Autodesk Inventor part; units mm, degrees
ref_plane "Work Plane2" through (300, 100, 0) normal (-0.9889364, -0.1483405, 0) x (0.1483405, -0.9889364, 0)
ref_plane "YZ Plane" through (0, 0, 0) normal (1, 0, 0) x (0, 1, 0)
ref_plane "XZ Plane" through (0, 0, 0) normal (0, 1, 0) x (-1, 0, 0)
sketch "Sketch1" plane through (0, 0, 0) normal (0, 0, 1) x (1, 0, 0)
  line L0 (-100, 0) -> (100, 0) construction
  line L1 (-100, 65) -> (-100, -65)
  circle A0 centre (-52.5, 57.5) radius 2.25
  line L2 (100, -70) -> (100, 70) construction
  line L3 (-92, 0) -> (-92, 57.5) construction
  line L4 (-92, 0) -> (-92, -57.5) construction
  circle A1 centre (-92.5, 57.5) radius 2.25
  circle A2 centre (-92.5, 57.5) radius 1.25
  circle A3 centre (-52.5, 57.5) radius 1.25
  line L5 (-100, 65) -> (-22.5777, 65)
  line L6 (-22.5777, 65) -> (-12.5777, 90)
  line L7 (-12.5777, 90) -> (100, 90)
  line L8 (100, 90) -> (100, 0)
  line L9 (100, -90) -> (100, 0)
  line L10 (-12.5777, -90) -> (100, -90)
  line L11 (-22.5777, -65) -> (-12.5777, -90)
  line L12 (-100, -65) -> (-22.5777, -65)
  line L13 (85, 75) -> (-2.4223, 75)
  line L14 (-2.4223, 75) -> (-12.4223, 50)
  line L15 (-12.4223, 50) -> (-92, 50)
  line L16 (-92, -50) -> (-12.4223, -50)
  line L17 (-12.4223, -50) -> (-2.4223, -75)
  line L18 (-2.4223, -75) -> (85, -75)
  line L19 (92.5, 82.5) -> (-7.5, 82.5) construction
  line L20 (-7.5, 82.5) -> (-17.5, 57.5) construction
  line L21 (-17.5, 57.5) -> (-92.5, 57.5) construction
  line L22 (-92.5, 57.5) -> (-92.5, -57.5) construction
  line L23 (-92.5, -57.5) -> (-17.5, -57.5) construction
  line L24 (-17.5, -57.5) -> (-7.5, -82.5) construction
  line L25 (-7.5, -82.5) -> (92.5, -82.5) construction
  line L26 (92.5, -82.5) -> (92.5, 0) construction
  line L27 (92.5, 0) -> (92.5, 82.5) construction
  line L28 (85, 75) -> (85, -75)
  line L29 (-100, 65) -> (-108, 65)
  line L30 (-108, 65) -> (-108, -65)
  line L31 (-108, -65) -> (-100, -65)
  line L32 (-100, -65) -> (-100, 65)
  line L33 (100, 0) -> (-108, 0)
  circle A4 centre (20, 82.5) radius 1.25
  circle A5 centre (20, 82.5) radius 2.25
  circle A6 centre (80, 82.5) radius 1.25
  circle A7 centre (80, 82.5) radius 2.25
  line L34 (50, 90) -> (50, 75) construction
  circle A8 centre (-12.5, 70) radius 1.25
  circle A9 centre (-12.5, 70) radius 2.25
  line L35 (-92, 50) -> (-92, -50)
  circle A10 centre (-96, 0) radius 2.25
  circle A11 centre (-96, 0) radius 1.25
  circle A12 centre (-104, 30) radius 2.25
  circle A13 centre (-104, 30) radius 1.25
  circle A14 centre (-104, -30) radius 2.25
  circle A15 centre (-104, -30) radius 1.25
  line L36 (-104, 65) -> (-104, -65) construction
  line L37 (-32, 50) -> (-32, 10)
  line L38 (-32, 10) -> (-92, 10)
  line L39 (77, 0) -> (77, -50)
  line L40 (77, -50) -> (-3, -50)
  line L41 (-3, -50) -> (-3, 0)
  line L42 (77, -40) -> (67, -40)
  line L43 (67, -40) -> (67, -50)
  line L44 (27, -50) -> (27, -40)
  line L45 (27, -40) -> (17, -40)
  line L46 (17, -40) -> (17, -50)
  circle A16 centre (57, 0) radius 7.5
  point P0 (0, 0)
  point P1 (0, 0)
  point P2 (77, 0)
  point P3 (-3, 0)
  dimension "d0" = 130
  dimension "d1" = 8
  dimension "d2" = 200
  dimension "d15" = 15
  dimension "d17" = 7.5
  dimension "d18" = 4.5
  dimension "d19" = 2.5
  dimension "d20" = 40
  dimension "d21" = 180
  dimension "d22" = 15
  dimension "d24" = 8
  dimension "d28" = 20
  dimension "d29" = 50
  dimension "d30" = 40
  dimension "d40" = 30
  dimension "d41" = 4
  dimension "d110" = 40
  dimension "d111" = 60
  dimension "d114" = 10
  dimension "d115" = 8
  dimension "d132" = 50
  dimension "d133" = 80
  dimension "d135" = 15
  dimension "d138" = 20
  dimension "d139" = 29
  dimension "d140" = 40
  dimension "d141" = 10
sketch "Sketch6" plane through (0, 0, 0) normal (0, 0, 1) x (1, 0, 0)
  line L0 (0, -140.4945) -> (0, 142.9668) construction
  line L1 (59.9258, 0) -> (340.445, 0) construction
  line L2 (100, -70) -> (100, 70) construction
  line L3 (300, -100) -> (100, -70)
  line L4 (300, 100) -> (100, 70)
  dimension "d146" = 300
  dimension "d147" = 100
ref_plane "Work Plane2" through (300, 100, 0) normal (-0.9889364, -0.1483405, 0) x (0.1483405, -0.9889364, 0)
sketch "Sketch7" plane through (300, 100, 0) normal (-0.9889364, -0.1483405, 0) x (0.1483405, -0.9889364, 0)
  circle A0 centre (0, 0) radius 2.5
  dimension "d150" = 5
extrude "Extrusion1" add sketch "Sketch1" along normal mid plane 94 contours L5 L6 L7 L8 L33 L28 L13 L14 L15 L35 A10 L1 | L1 L33 L30 L29 | L33 A10 L35 L16 L17 L18 L28 L9 L10 L11 L12 L1 | L1 L31 L30 L33 | A10 L33 A11 | L33 A11 A10 | A11 L33 | L33 A11 | L35 L38 L37 L15 L14 L13 L28 L33 A16 | L33 L41 L40 L39 L28 L18 L17 L16 L35 | L33 A16 L39 L42 L43 L40 L44 L45 L46 L41 | L35 L15 L37 L38 | A16 L33 | L33 A16 | L46 L45 L44 L40 | L39 L40 L43 L42 | A0 | A1 | A2 | A3 | A4 | A5 | A6 | A7 | A8 | A9 | A12 | A13 | A14 | A15
extrude "Extrusion2" cut sketch "Sketch1" along normal mid plane 59 contours L35 L38 L37 L15 L14 L13 L28 L33 A16 | L33 L41 L40 L39 L28 L18 L17 L16 L35 | L33 A16 L39 L42 L43 L40 L44 L45 L46 L41 | L35 L15 L37 L38 | A16 L33 | L33 A16 | L46 L45 L44 L40 | L39 L40 L43 L42
sketch "Sketch2" plane through (-108, -65, 47) normal (-1, 0, 0) x (0, 0, 1)
  line L0 (0, -25) -> (0, 155)
  line L1 (-94, 15) -> (0, 15)
  line L2 (0, 15) -> (0, 115)
  line L3 (0, 115) -> (-94, 115)
  line L4 (-94, 115) -> (-94, 15)
  line L5 (-94, 15) -> (0, 115) construction
  line L6 (0, 15) -> (-94, 115) construction
  line L7 (-94, 42) -> (0, 42)
  line L8 (0, 42) -> (0, 88)
  line L9 (0, 88) -> (-94, 88)
  line L10 (-94, 88) -> (-94, 42)
  line L11 (-94, 42) -> (0, 88) construction
  line L12 (0, 42) -> (-94, 88) construction
  point P0 (-47, 65)
  dimension "d52" = 100
  dimension "d55" = 46
extrude "Extrusion3" add sketch "Sketch2" along normal blind 88
extrude "Extrusion4" [suppressed]
sketch "Sketch3" plane through (0, 0, 0) normal (0, 1, 0) x (-1, 0, 0)
  circle A0 centre (153, 0) radius 32.5
  line L0 (108, -47) -> (108, 47)
  line L1 (108, -47) -> (108, 47)
  line L2 (108, -47) -> (108, 47) construction
  line L3 (108, 0) -> (245.8238, 0) construction
  circle A1 centre (153, 0) radius 40
  line L4 (183.942, 9.942) -> (196, 22)
  line L5 (196, 22) -> (196, -22)
  line L6 (196, -22) -> (183.942, -9.942)
  line L7 (196, 47) -> (196, -47)
  line L8 (204, 47) -> (224, 20)
  line L9 (224, 20) -> (224, 47)
  line L10 (224, 47) -> (204, 47)
  line L11 (196, -47) -> (224, -47)
  line L12 (204, -47) -> (224, -20)
  line L13 (224, -20) -> (224, -47)
  line L14 (-100, 47) -> (12.5777, 47)
  line L15 (-100, 47) -> (-100, 32)
  line L16 (-100, 32) -> (-90, 47)
  line L17 (-100, -47) -> (12.5777, -47)
  line L18 (-100, -47) -> (-100, -32)
  line L19 (-100, -32) -> (-90, -47)
  circle A2 centre (-48, 0) radius 46
  line L20 (-100, 47) -> (-100, -47)
  circle A3 centre (-48, 0) radius 32.5
  line L21 (-4.8723, -16) -> (13.1277, -16)
  line L22 (13.1277, -16) -> (13.1277, 16)
  line L23 (13.1277, 16) -> (-4.8723, 16)
  point P0 (0, 0)
  point P1 (189.7631, 15.7631)
  point P2 (189.7631, -15.7631)
  dimension "d58" = 45
  dimension "d59" = 65
  dimension "d62" = 80
  dimension "d64" = 44
  dimension "d69" = 20
  dimension "d70" = 27
  dimension "d80" = 15
  dimension "d81" = 10
  dimension "d87" = 52
  dimension "d88" = 92
  dimension "d116" = 65
  dimension "d121" = 32
  dimension "d122" = 18
  dimension "d134" = 8
  dimension "d143" = 48
extrude "Extrusion15" cut sketch "Sketch3" along normal through all both and the other way through all contours L10 L9 L8 | L12 L13 L11 | L14 L16 L15 | L18 L19 L17
extrude "Extrusion16" add sketch "Sketch1" along normal through all both and the other way through all contours L35 L15 L37 L38
extrude "Extrusion14" add sketch "Sketch3" against normal blind 32 from surface at -90 contours A2 | A3
extrude "Extrusion17" [suppressed]
extrude "Extrusion18" cut sketch "Sketch3" along normal blind 5 from surface at -50 contours A0
extrude "Extrusion21" cut sketch "Sketch1" along normal up to surface (17.5 mm away) from surface at -47 contours A16 L33 | L33 A16
extrude "Extrusion22" add sketch "Sketch1" along normal blind 30 from surface at -29.5 contours L33 A16 L39 L42 L43 L40 L44 L45 L46 L41 | L33 A16 | L46 L45 L44 L40 | L39 L40 L43 L42 picked at (58.4928, -2.6557)
extrude "Extrusion24" [suppressed]
mirror "Mirror2" about plane through (0, 0, 0) normal (0, 1, 0) of "Extrusion14", "Extrusion16", "Extrusion18", "Extrusion22"
equation "\"d17\" = 0.5 * d15"
equation "\"d21\" = d47"
equation "\"d45\" = 124"
equation "\"d46\" = 12"
equation "\"d47\" = 180"
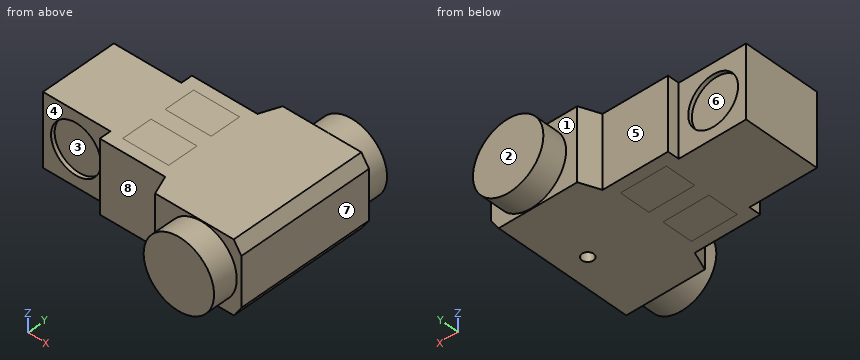
Geometry: final body of the model. Coordinates: model frame, mm. Face numbers are marked on the shaded views. A direction names the side the tool comes from. Give positions to 0.01 mm unless a question says otherwise; leave off trailing zeros. Loops run counter-clockwise (first coordinate to the right, second up) from the corner with the lowest first, then second, coordinate; pieces in that order, holes last. Notation, with made-up numbers: (54, -32.5) - (107, -32.5) arc R30 cw to (107, 3.5) - close; hole circle Ø7 at (64.25, 20.25). An arc over 180 degrees is marked (long way). One line per question, with ' | ' between items. Start each with the question number.
(1) Section query D-D on x = -153. Return loops of the section in (y, z), then the cut area to 3 significant figures.
(2) Section query C-C on z = -15. Count the separate pieces of the cut face and the enclosed holes in it, then the cut area to 3 significant figures.
(3) Section query B-B on y = 0. Return loops of the section in (x, z).
(4) Section query A-A on x = -42. Return loops of the section in (y, z), then the cut area to 3 significant figures.
(5) Contact query for flat-ended pins moving along their axis: pin 1 (6 mm diameter, centred on y = -66.5, z = 29.5, fed in from -X); pin 2 (2 mm diameter, centred on y = 95.5, z = -19.5, fed in from -X); pin 3 (13.5 mm diameter, centred on x = 57, y = 0, fed in from -Z). Output: stop coordinate, or through.
(6) Pull-direction query (X, two-part tool) for the marked faces 6, 7 and 8; classes: released by +X, released by -X, zero draft, split by the parting line, or undercut.
(7) Ray query, line 1 (Y direction, x = -27, z = 21); line 2 (Z direction, x = -153, y = -46.7); line 3 (Z direction, x = 7.5, y = -32.5). Return the intervals inside material, ascending. Write a range as from..to.
(8) Reachability of the marked faces 1, 2, 3, 4 and 5 from +Z, -Z, +X, -X, +Y, -Y: full face, straight path, thin tool, end or side. Return the list, or none.
The answers:
1) outline: (-50, -47) - (50, -47) - (50, -32.5) - (45, -32.5) - (45, 32.5) - (50, 32.5) - (50, 47) - (-50, 47) - (-50, 32.5) - (-45, 32.5) - (-45, -32.5) - (-50, -32.5) - close | area: 8,750 mm2
2) separate pieces: 2 | enclosed holes: 1 | area: 37,200 mm2
3) outline: (-196, -47) - (49.5, -47) - (49.5, -29.5) - (64.5, -29.5) - (64.5, -47) - (90, -47) - (100, -32) - (100, 32) - (90, 47) - (-196, 47) - close; hole (-92, -29.5) - (-3, -29.5) - (-3, 0.5) - (77, 0.5) - (77, -29.5) - (85, -29.5) - (85, 29.5) - (-92, 29.5) - close
4) outline: (-65, -47) - (-50, -47) - (65, -47) - (65, 47) - (10, 47) - (-50, 47) - (-65, 47) - close; hole (-10, -29.5) - (10, -29.5) - (10, 29.5) - (-10, 29.5) - close | area: 11,000 mm2
5) pin 1: x = -108 | pin 2: x = 5.88 | pin 3: z = -29.5
6) face 6: undercut | face 7: released by +X | face 8: zero draft
7) line 1: -65..-50, 50..65 | line 2: -47..-32.5, 32.5..47 | line 3: -47..0.5, 29.5..47
8) face 1: +Y | face 2: +Z, -Z, +X, -X, +Y | face 3: -Y | face 4: +Z, -Z, -X, -Y | face 5: +Z, -Z, -X, +Y
